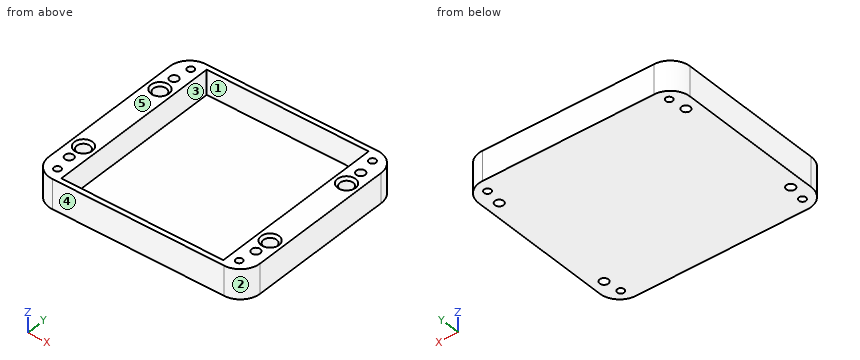
```python
from build123d import *

# Parameters (mm, degrees)
F1_DEPTH = 2
F2_R     = 2.65
F2_W     = 65.6
F2_H     = 71.7
F3_DEPTH = 10
F4_R     = 1.4
F4_R_2   = 1.75
F5_DEPTH = 12
F6_SIZE  = 1


with BuildPart() as f1:
    # F0 (on Top) → F1 (new body)
    with BuildSketch(Plane.XY):
        with BuildLine():
            Line((34.8, 37.85), (-34.8, 37.85))
            ThreePointArc((-34.8, 37.85), (-40.456854, 35.506854), (-42.8, 29.85))
            Line((-42.8, 29.85), (-42.8, -29.85))
            ThreePointArc((-42.8, -29.85), (-40.456854, -35.506854), (-34.8, -37.85))
            Line((-34.8, -37.85), (34.8, -37.85))
            ThreePointArc((34.8, -37.85), (40.456854, -35.506854), (42.8, -29.85))
            Line((42.8, -29.85), (42.8, 29.85))
            ThreePointArc((42.8, 29.85), (40.456854, 35.506854), (34.8, 37.85))
        make_face()
    extrude(amount=F1_DEPTH)

    # F2 (on face) → F3 (join)
    with BuildSketch(Plane.XY.offset(2)):
        with BuildLine():
            ThreePointArc((-34.8, 37.85), (-40.456854, 35.506854), (-42.8, 29.85))
            Line((-42.8, 29.85), (-42.8, -29.85))
            ThreePointArc((-42.8, -29.85), (-40.456854, -35.506854), (-34.8, -37.85))
            Line((-34.8, -37.85), (34.8, -37.85))
            ThreePointArc((34.8, -37.85), (40.456854, -35.506854), (42.8, -29.85))
            Line((42.8, -29.85), (42.8, 29.85))
            ThreePointArc((42.8, 29.85), (40.456854, 35.506854), (34.8, 37.85))
            Line((34.8, 37.85), (-34.8, 37.85))
        make_face()
        with Locations((-37.8, -18.85)):
            Circle(F2_R, mode=Mode.SUBTRACT)
        with Locations((37.8, -18.85)):
            Circle(F2_R, mode=Mode.SUBTRACT)
        with Locations((-37.8, 18.85)):
            Circle(F2_R, mode=Mode.SUBTRACT)
        Rectangle(F2_W, F2_H, mode=Mode.SUBTRACT)
        with Locations((37.8, 18.85)):
            Circle(F2_R, mode=Mode.SUBTRACT)
    extrude(amount=F3_DEPTH)

    # F4 (on face) → F5 (cut, through all)
    with BuildSketch(Plane.XY.offset(12)):
        with Locations((-36.8, -32.85)):
            Circle(F4_R)
        with Locations((36.8, -32.85)):
            Circle(F4_R)
        with Locations((-36.8, 32.85)):
            Circle(F4_R)
        with Locations((36.8, 32.85)):
            Circle(F4_R)
        with Locations((-37.8, -25.85)):
            Circle(F4_R_2)
        with Locations((37.8, -25.85)):
            Circle(F4_R_2)
        with Locations((-37.8, 25.85)):
            Circle(F4_R_2)
        with Locations((37.8, 25.85)):
            Circle(F4_R_2)
    extrude(amount=-F5_DEPTH, mode=Mode.SUBTRACT)

    # F6
    f6_edges = [f1.edges().sort_by_distance(p)[0] for p in [
        (-40.45, 18.85, 12),
        (35.15, 18.85, 12),
        (35.15, -18.85, 12),
        (-40.45, -18.85, 12),
    ]]
    chamfer(f6_edges, length=F6_SIZE)


solid = f1.part
```
Design review of the part built by this model. Coordinates are the model's own, in mm. Face numbers are marked on the shaded views. A direction names the side the tool comes from. Round coordinates to 2 decimals unless told otherwise and drop trailing zeros. Write each loop counter-clockwise with the first axis right and the second up, starting at its lowest first coordinate (ties: lowest second). Pieces come first, ordered by that corner, then holes. Notation, with made-up numbers: (89, -36.75) -> (115, -36.75) arc R17 ccw to (115, -3.75) -> close; hole circle Ø4 at (-5, 57.25). An arc over 180 degrees is marked (long way). Write item = value, one per line. Start each with the question number.
1) Tool access review of the marked faces 1 and 2: name each direction out of +Z, -Z, +X, -X, +Y, -Y from which nothing blocks a thin tool from reaching the whole face with its end or side.
2) Take a section at C-C, the plane x = 26. State the section outline as (y, z) points.
3) Take a section at B-B, the plane z = 9.5. Count the separate pieces of the cut face and the enclosed holes in it, plus the area to 3 significant figures.
4) Take a section at A-A, the plane y = 25.85. State the section outline as (x, z) points.
5) Wall thickness on probe 1 along X at (y, z) = (3, 4.25); probe 2 along Y at (x, z) = (22.5, 2.5); probe 3 along X at (y, z) = (17.5, 10.25): over which ranges is each line inside the solid? List them lowest first. Write a range as from..to.
6) Mouldability with a two-part tool opening along Y and no side actions: class the marked faces 3, 4 and 5 as +Y half, -Y half, draft (parallel to the pull), parting line (faces both ways), or undercut.
7) Take a section at D-D, the plane y = 0. State the section outline as (x, z) points.
8) Clearance check with flat-ended pins moving along their axes: pin 1 (1.6 mm diameter, centred on x = -38.5, y = 18, fed in from +Z); pin 2 (12 mm diameter, centred on x = 27, y = 22.5, fed in from -Z); pin 3 (6 mm diameter, centred on x = -37.8, y = 18.85, fed in from +Z). State where each tip first meets the part, or that it passes through.
Results list:
q1.face_1 = +Z
q1.face_2 = +Z, -Z, +X, -Y
q2.outline = (-37.85, 0) -> (37.85, 0) -> (37.85, 12) -> (35.85, 12) -> (35.85, 2) -> (-35.85, 2) -> (-35.85, 12) -> (-37.85, 12) -> close
q3.separate_pieces = 1
q3.enclosed_holes = 13
q3.area = 1,570 mm²
q4.outline = (-42.8, 0) -> (-39.55, 0) -> (-39.55, 12) -> (-42.8, 12) -> close; (-36.05, 0) -> (36.05, 0) -> (36.05, 12) -> (32.8, 12) -> (32.8, 2) -> (-32.8, 2) -> (-32.8, 12) -> (-36.05, 12) -> close; (39.55, 0) -> (42.8, 0) -> (42.8, 12) -> (39.55, 12) -> close
q5.probe_1 = -42.8..-32.8, 32.8..42.8
q5.probe_2 = -37.85..-35.85, 35.85..37.85
q5.probe_3 = -42.8..-40.08, -35.52..-32.8, 32.8..35.52, 40.08..42.8
q6.face_3 = undercut
q6.face_4 = -Y half
q6.face_5 = draft
q7.outline = (-42.8, 0) -> (42.8, 0) -> (42.8, 12) -> (32.8, 12) -> (32.8, 2) -> (-32.8, 2) -> (-32.8, 12) -> (-42.8, 12) -> close
q8.pin_1 = 2
q8.pin_2 = 0
q8.pin_3 = 11.35
